Here's how the part is built. I have some questions about the finished solid (model axes, mm). Face numbers are marked on the shaded views. A direction names the side the tool comes from. Coordinates: 2 decimals unless noted, no trailing zeros. Write each loop counter-clockwise with the first axis right and the second up, starting at its lowest first coordinate (ties: lowest second). Pieces come first, ordered by that corner, then holes. Notation, with made-up numbers: (66.25, 3) -> (116.25, 3) arc R5 cw to (116.25, 9) -> close; hole circle Ø7 at (76.25, -31). An arc over 180 degrees is marked (long way). Answer in a Markdown table with one row per item. Add a question column.
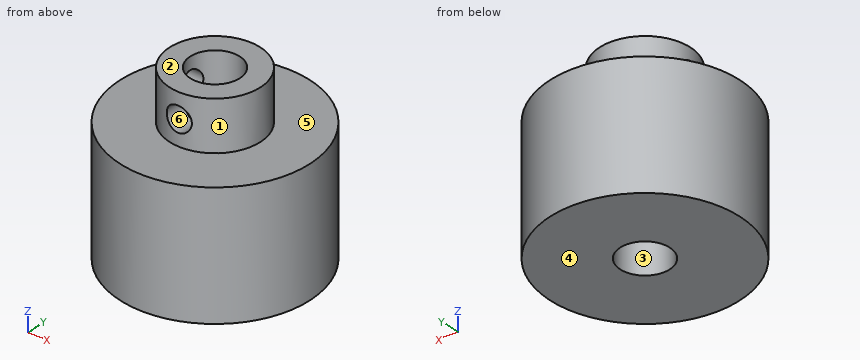
from build123d import *

# Parameters (mm, degrees)
SKETCH1_R           = 11.5
BOSS_EXTRUDE1_DEPTH = 15
SKETCH2_R           = 5.5
BOSS_EXTRUDE2_DEPTH = 6
SKETCH3_R           = 3
CUT_EXTRUDE1_DEPTH  = 27.561249971
SKETCH4_R           = 1.5
CUT_EXTRUDE2_DEPTH  = 27.561249971
SKETCH5_R           = 1.5
CUT_EXTRUDE3_DEPTH  = 27.56125005


with BuildPart() as part:
    # Sketch1 → Boss-Extrude1 (new body)
    with BuildSketch(Plane.XY):
        Circle(SKETCH1_R)
    extrude(amount=BOSS_EXTRUDE1_DEPTH)

    # Sketch2 → Boss-Extrude2 (add)
    with BuildSketch(Plane.XY.offset(15)):
        Circle(SKETCH2_R)
    extrude(amount=BOSS_EXTRUDE2_DEPTH)

    # Sketch3 → Cut-Extrude1 (cut, through all)
    with BuildSketch(Plane.XY.offset(21)):
        Circle(SKETCH3_R)
    extrude(amount=-CUT_EXTRUDE1_DEPTH, mode=Mode.SUBTRACT)

    # Sketch4 → Cut-Extrude2 (cut, through all)
    with BuildSketch(Plane(origin=(0, 0, 0), x_dir=(1, 0, 0), z_dir=(0, 1, 0))):
        with Locations(Location((0, -18, 0), (0, 0, 270))):
            Circle(SKETCH4_R)
    extrude(amount=-CUT_EXTRUDE2_DEPTH, mode=Mode.SUBTRACT)

    # Sketch5 → Cut-Extrude3 (cut, through all)
    with BuildSketch(Plane(origin=(0, 0, 0), x_dir=(0, 0, -1), z_dir=(1, 0, 0))):
        with Locations((-18, 0)):
            Circle(SKETCH5_R)
    extrude(amount=-CUT_EXTRUDE3_DEPTH, mode=Mode.SUBTRACT)


solid = part.part
Q1. I need wall thicknesses on line 1 (Z direction, x = 0, y = -4.6); line 2 (Z direction, x = -9.5, y = -3); line 3 (X direction, y = -1.5, z = 4.25). Which ranges of each line are inside material? Lowest first, please. Write a range as [from, to].
Q2. Imagine slicing it at A-A on y = 0. Please give me the cut outline in (x, z), plus the area to 4 significant figures.
Q3. If we mould it in two halves opening along X, with no side actions, what happens to the marked faces 1, 2 and 3? For each: pulls with the +X half, pulls with the -X half, needs draft (parallel to the pull), parting line crosses it, or undercut.
Q4. Imagine slicing it at C-C on z = 18. Please give me the cut outline in (x, y).
Q5. I'm going to push flat-ended pins straight in: P1, Ø1.5, axis at y = 4.5, z = 13, coming from the -X side; P2, Ø4, axis at y = -3.5, z = 18.5, coming from the +X side; P3, Ø1, axis at x = -1.5, z = 19, coming from the +Y side; P4, Ø5, axis at x = 0, y = 0, coming from the -Z side. Where does each tip first touch, or does it pass through?
Q6. For the marked faces 4, 5 and 6, which set-ups out of +Z, -Z, +X, -X, +Y, -Y let a thin tool reach every point of the face, with its end or its side?
Q7. Imagine slicing it at D-D on y = -3.75. Please give me the cut outline in (x, z), plus the area to 3 significant figures.
Result sheet:
| question | item | result |
|---|---|---|
| 1 | line 1 | z = [0, 16.5], [19.5, 21] |
| 1 | line 2 | z = [0, 15] |
| 1 | line 3 | x = [-11.4, -2.6], [2.6, 11.4] |
| 2 | outline | (-11.5, 0) -> (-3, 0) -> (-3, 16.5) -> (-5.5, 16.5) -> (-5.5, 15) -> (-11.5, 15) -> close; (-5.5, 19.5) -> (-3, 19.5) -> (-3, 21) -> (-5.5, 21) -> close; (3, 0) -> (11.5, 0) -> (11.5, 15) -> (5.5, 15) -> (5.5, 21) -> (3, 21) -> close |
| 2 | area | 277.5 mm^2 |
| 3 | face 1 | parting line crosses it |
| 3 | face 2 | needs draft |
| 3 | face 3 | undercut |
| 4 | outline | (-5.29, -1.5) arc R5.5 ccw to (-1.5, -5.29) -> (-1.5, -2.6) arc R3 cw to (-2.6, -1.5) -> close; (-5.29, 1.5) -> (-2.6, 1.5) arc R3 cw (long way) to (1.5, -2.6) -> (1.5, -5.29) arc R5.5 ccw (long way) to start |
| 5 | P1 | stops at x = -10.87 |
| 5 | P2 | stops at x = 5.29 |
| 5 | P3 | stops at y = 5.41 |
| 5 | P4 | passes through |
| 6 | face 4 | -Z, +X, -X, +Y, -Y |
| 6 | face 5 | +Z |
| 6 | face 6 | -Y |
| 7 | outline | (-10.87, 0) -> (10.87, 0) -> (10.87, 15) -> (4.02, 15) -> (4.02, 21) -> (-4.02, 21) -> (-4.02, 15) -> (-10.87, 15) -> close; hole circle Ø3 at (0, 18) |
| 7 | area | 367 mm^2 |
